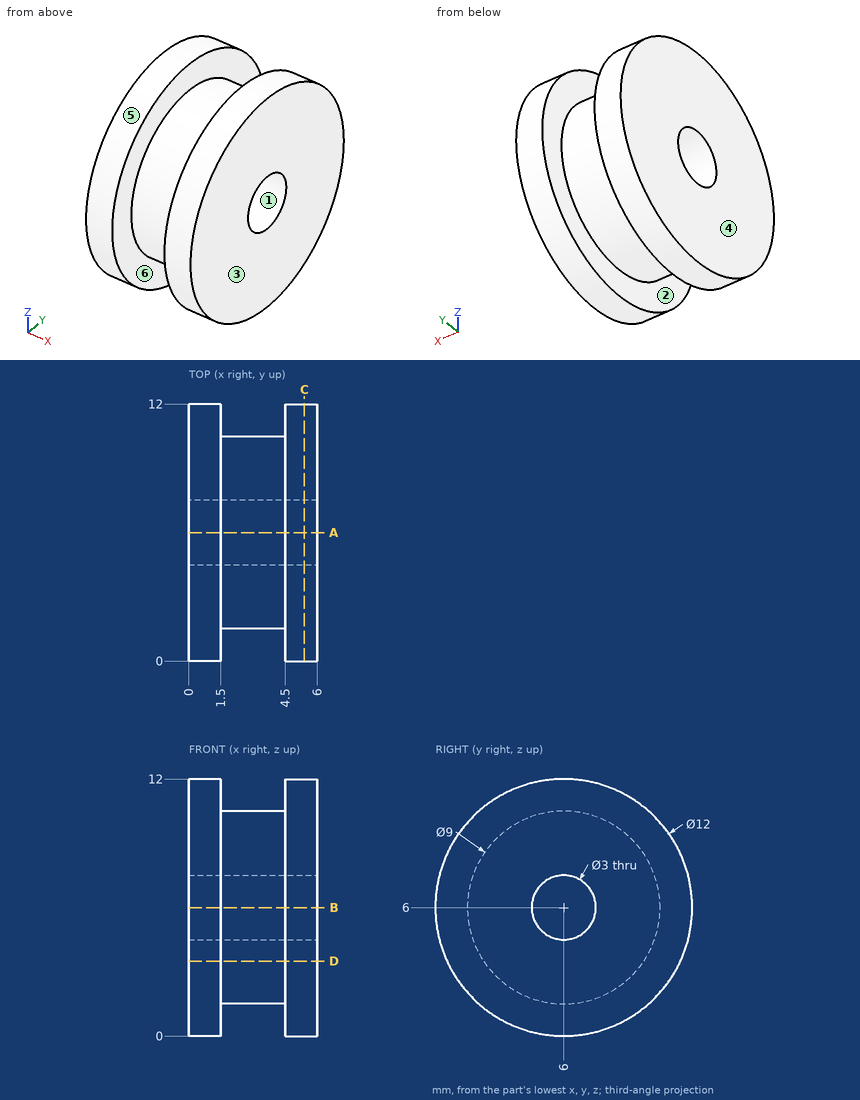
Can you work these out from the drawing? Everything is in mm from the part's minimum corner. A direction names the side the tool comes from. Round coordinates to 2 decimals unless told otherwise and drop trailing zeros. Write each loop counter-clockwise with the first axis right and the second up, starting at its lowest first coordinate (ties: lowest second). Pieces come first, ordered by that corner, then holes.
1. Suppose I cut it at A-A (y = 6). List the corners of the cut face in (x, z) for me.
2. I need wall thicknesses on L1, parallel to X at y = 8, z = 10.25; L2, parallel to Z at x = 1.75, y = 6; L3, parallel to Z at x = 0.3, y = 5.5. Which ranges of each line are inside material? Lowest first, please.
3. If we mould it in two halves opening along X, with no side actions, what happens to the marked faces 1, 2, 3 and 4? For each: released by +X, released by -X, zero draft, split by the parting line, or undercut.
4. Suppose I cut it at C-C (x = 5.4). List the corners of the cut face in (y, z) for me, and give its area (3 significant figures).
5. Will these pins go through, and if not, where does the flat tip stop? pin 1 Ø3.5 at (y, z) = (4, 4.5) entering from -X; pin 2 Ø2 at (x, y) = (0.5, 3.5) entering from +Z; pin 3 Ø1.5 at (x, y) = (5, 4.5) entering from -Z.
6. For the marked faces 5 and 6, which set-ups out of +Z, -Z, +X, -X, +Y, -Y let a thin tool reach every point of the face, with its end or its side?
7. Suppose I cut it at D-D (z = 3.5). List the corners of the cut face in (x, y) for me, and give its area (3 significant figures).
Answer sheet:
1. outline: (0, 0) - (1.5, 0) - (1.5, 1.5) - (4.5, 1.5) - (4.5, 0) - (6, 0) - (6, 4.5) - (0, 4.5) - close; (0, 7.5) - (6, 7.5) - (6, 12) - (4.5, 12) - (4.5, 10.5) - (1.5, 10.5) - (1.5, 12) - (0, 12) - close
2. L1: x = 0 to 1.5, 4.5 to 6
2. L2: z = 1.5 to 4.5, 7.5 to 10.5
2. L3: z = 0.02 to 4.59, 7.41 to 11.98
3. face 1: zero draft
3. face 2: undercut
3. face 3: released by +X
3. face 4: released by -X
4. outline: circle Ø12 at (6, 6); hole circle Ø3 at (6, 6)
4. area: 106 mm2
5. pin 1: stops at x = 0
5. pin 2: stops at z = 11.81
5. pin 3: stops at z = 0.05
6. face 5: +X, -X
6. face 6: none
7. outline: (0, 0.55) - (1.5, 0.55) - (1.5, 2.26) - (4.5, 2.26) - (4.5, 0.55) - (6, 0.55) - (6, 11.45) - (4.5, 11.45) - (4.5, 9.74) - (1.5, 9.74) - (1.5, 11.45) - (0, 11.45) - close
7. area: 55.2 mm2
